For this review, take the finished solid that the model builds, in its own axes (mm). Face numbers are marked on the shaded views. Coordinates: 2 decimals unless noted, no trailing zeros. Write each loop counter-clockwise with the first axis right and the second up, starting at its lowest first coordinate (ties: lowest second). Pieces come first, ordered by that corner, then holes.
```python
from build123d import *

# Parameters (mm, degrees)
F1_DEPTH = 127
F2_R     = 11.1125
F3_DEPTH = 127
F4_R     = 11.132084
F5_DEPTH = 409.90812


with BuildPart() as f1:
    # F0 (on Front) → F1 (new body)
    with BuildSketch(Plane.XZ):
        with BuildLine():
            Line((12.7, 0), (-12.7, 0))
            ThreePointArc((-12.7, 0), (0, -12.7), (12.7, 0))
        make_face()
    extrude(amount=F1_DEPTH)

    # F2 (on Front) → F3 (join)
    with BuildSketch(Plane.XZ):
        Circle(F2_R)
    extrude(amount=F3_DEPTH)

    # F4 (on face) → F5 (cut)
    with BuildSketch(Plane(origin=(0, 0, 0), x_dir=(-1, 0, 0), z_dir=(0, 1, 0))):
        Circle(F4_R)
    extrude(amount=-F5_DEPTH, mode=Mode.SUBTRACT)


solid = f1.part
```
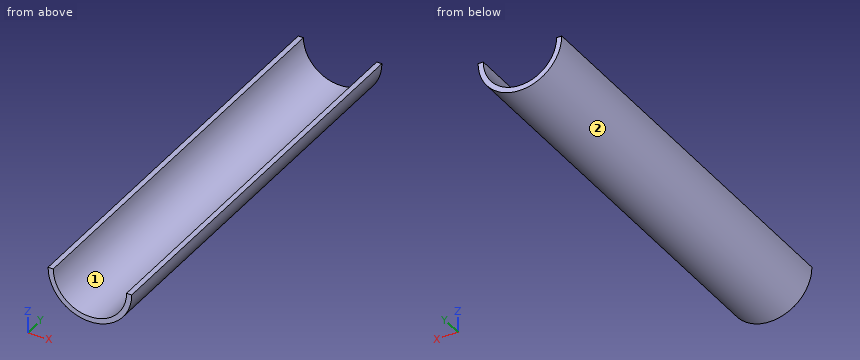
Q1. Add section A-A (z = -10). State the section outline as (x, y) points.
Ans:
outline: (-7.83, -127) - (-4.89, -127) - (-4.89, 0) - (-7.83, 0) - close; (4.89, -127) - (7.83, -127) - (7.83, 0) - (4.89, 0) - close
Q2. Add section B-B (x = 0). State the section outline as (y, z) points.
Ans:
outline: (-127, -12.7) - (0, -12.7) - (0, -11.13) - (-127, -11.13) - close
Q3. Draft analysis for pull direction X (two halves, no side actions). For the marked faces 1 and 2, state which applies: +X half, -X half, draft (parallel to the pull), parting line (faces both ways), or undercut.
Ans:
face 1: undercut
face 2: parting line
Q4. Add section D-D (z = -4.5). State the section outline as (x, y) points, then the cut area to 3 significant figures.
Ans:
outline: (-11.88, -127) - (-10.18, -127) - (-10.18, 0) - (-11.88, 0) - close; (10.18, -127) - (11.88, -127) - (11.88, 0) - (10.18, 0) - close
area: 430 mm2
Q5. Add section C-C (y = -90). State the section outline as (x, z) points.
Ans:
outline: (-12.7, 0) arc R12.7 ccw to (12.7, 0) - (11.13, 0) arc R11.13 cw to (-11.13, 0) - close
Q6. For probe 1 along X at (y, z) = (-111, -10); probe 2 along X at (y, z) = (-12, -6); probe 3 along Z at (x, y) = (-9.5, -100), list the stretches that pass through material, from the lowest coordinate up.
Ans:
probe 1: x = -7.83 to -4.89, 4.89 to 7.83
probe 2: x = -11.19 to -9.38, 9.38 to 11.19
probe 3: z = -8.43 to -5.8
Q7. Clearance check with flat-ended pins moving along their axes: pin 1 Ø4 at (y, z) = (-101, -4.5) entering from +X; pin 2 Ø6 at (y, z) = (-69.5, -8) entering from +X; pin 3 Ø8 at (x, y) = (3.5, -74) entering from +Z. State where each tip first meets the part, or that it passes through.
Ans:
pin 1: stops at x = 12.45
pin 2: stops at x = 11.67
pin 3: stops at z = -8.23
